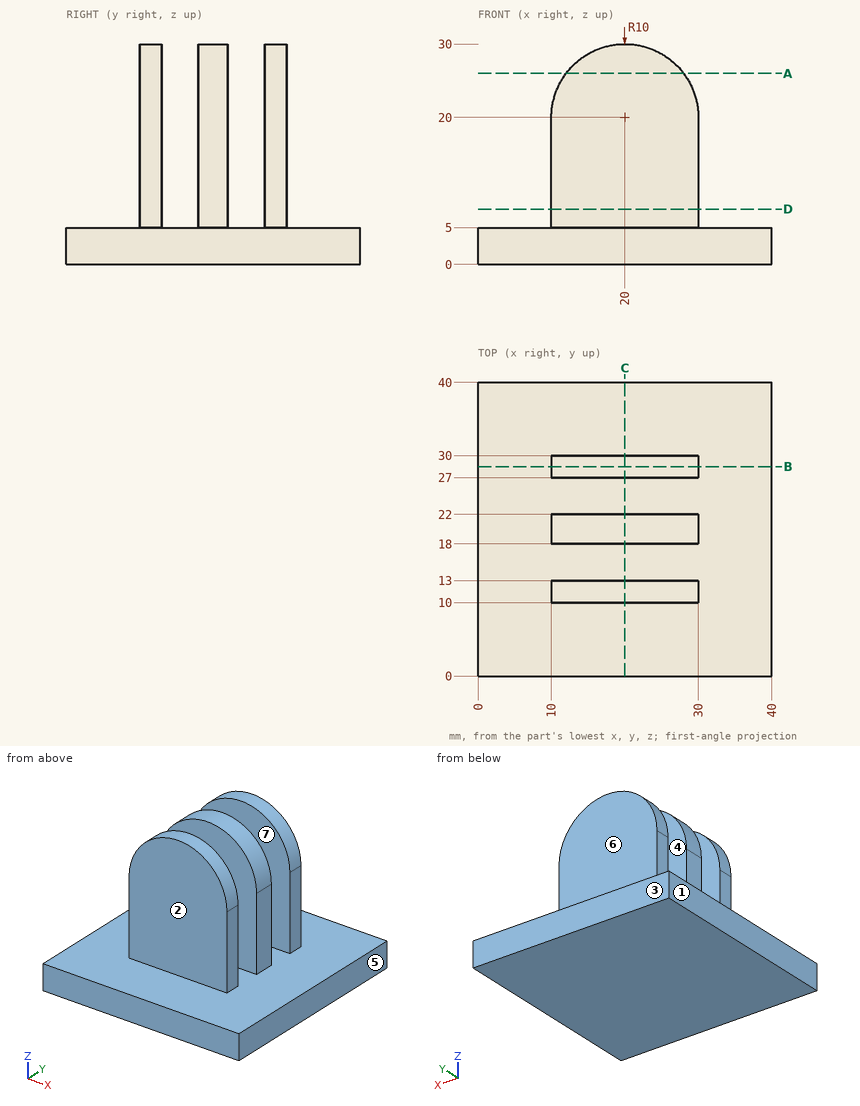
Could you check a few things on this drawing? It's one solid part, dimensions in mm from its lowest x, y, z. A direction names the side the tool comes from. Give positions to 0.01 mm unless a question says otherwise; leave off trailing zeros. Order: outer loops, then holes, each group sorted by start corner. A loop starts at its lowest first (then second) coordinate and runs counter-clockwise, first axis right, second up. Notation, with made-up numbers: (49.5, -11) -> (82.5, -11) arc R33 ccw to (82.5, 28) -> close; hole circle Ø5 at (-4.5, 27). An arc over 180 degrees is marked (long way). Answer in a Markdown table with one row per item. Add a question column.
Item 1: Imagine slicing it at D-D (z = 7.5). List the corners of the cut face in (x, y) for me.
Item 2: Imagine slicing it at A-A (z = 26). List the corners of the cut face in (x, y) for me, and give its area (3 significant figures).
Item 3: I'm going to push flat-ended pins straight in: P1, Ø8, axis at x = 28.5, z = 19.5, coming from the -Y side; P2, Ø1.5, axis at y = 18.5, z = 16, coming from the +X side; P3, Ø6, axis at y = 26.5, z = 17, coming from the -X side. Where does each tip first touch, or does it pass through?
Item 4: Imagine slicing it at B-B (y = 28.5). List the corners of the cut face in (x, z) for me, and give its area (3 significant figures).
Item 5: For the marked faces 5, 6 and 7, which set-ups out of +Z, -Z, +X, -X, +Y, -Y let a thin tool reach every point of the face, with its end or its side?
Item 6: We'd pull the mould along Y, two halves only. Please class the marked faces 1, 2, 3 and 4: pulls with the +Y half, pulls with the -Y half, needs draft (parallel to the pull), parting line crosses it, or undercut.
Item 7: Please list where these lines run through material, in increasing order: probe 1 along Y at (x, z) = (25.5, 12); probe 2 along Z at (x, y) = (11.5, 24.5); probe 3 along X at (y, z) = (18.5, 5.5).
Item 8: Imagine slicing it at C-C (x = 20). List the corners of the cut face in (y, z) for me.
Result:
| question | item | result |
|---|---|---|
| 1 | outline | (10, 10) -> (30, 10) -> (30, 13) -> (10, 13) -> close; (10, 18) -> (30, 18) -> (30, 22) -> (10, 22) -> close; (10, 27) -> (30, 27) -> (30, 30) -> (10, 30) -> close |
| 2 | outline | (12, 10) -> (28, 10) -> (28, 13) -> (12, 13) -> close; (12, 18) -> (28, 18) -> (28, 22) -> (12, 22) -> close; (12, 27) -> (28, 27) -> (28, 30) -> (12, 30) -> close |
| 2 | area | 160 mm2 |
| 3 | P1 | y = 10 |
| 3 | P2 | x = 30 |
| 3 | P3 | x = 10 |
| 4 | outline | (0, 0) -> (40, 0) -> (40, 5) -> (30, 5) -> (30, 20) arc R10 ccw to (10, 20) -> (10, 5) -> (0, 5) -> close |
| 4 | area | 657 mm2 |
| 5 | face 5 | +Z, -Z, +X, +Y, -Y |
| 5 | face 6 | +Z, +X, -X, +Y |
| 5 | face 7 | +Z, +X, -X |
| 6 | face 1 | needs draft |
| 6 | face 2 | pulls with the -Y half |
| 6 | face 3 | pulls with the +Y half |
| 6 | face 4 | undercut |
| 7 | probe 1 | 10 to 13, 18 to 22, 27 to 30 |
| 7 | probe 2 | 0 to 5 |
| 7 | probe 3 | 10 to 30 |
| 8 | outline | (0, 0) -> (40, 0) -> (40, 5) -> (30, 5) -> (30, 30) -> (27, 30) -> (27, 5) -> (22, 5) -> (22, 30) -> (18, 30) -> (18, 5) -> (13, 5) -> (13, 30) -> (10, 30) -> (10, 5) -> (0, 5) -> close |
